```python
from build123d import *

# Parameters (mm, degrees)
SKETCH_1_W          = 55
SKETCH_1_H          = 40
EXTRUDE_1_DEPTH     = 13
SHELL_1_T           = -1
CHAMFER_1_SIZE      = 1
CUT_EXTRUDE_3_DEPTH = 2
EXTRUDE_5_DEPTH     = 12
SKETCH_16_W         = 5
SKETCH_16_H         = 11
CUT_EXTRUDE_4_DEPTH = 1
SKETCH_18_W         = 8
SKETCH_18_H         = 8
CUT_EXTRUDE_5_DEPTH = 10
SKETCH_19_W         = 1
SKETCH_19_H         = 8
EXTRUDE_6_DEPTH     = 1
SKETCH_21_W         = 0.2
SKETCH_21_H         = 1
CUT_EXTRUDE_6_DEPTH = 12
SKETCH_20_W         = 1.5
SKETCH_20_H         = 10
EXTRUDE_8_DEPTH     = 17.5
EXTRUDE_9_DEPTH     = 10
SKETCH_7_R          = 1
EXTRUDE_4_DEPTH     = 3
FILLET_1_R          = 2
FILLET_2_R          = 0.3
FILLET_3_R          = 0.3


with BuildPart() as part:
    # 草图1 → 凸台-拉伸1 (new body)
    with BuildSketch(Plane(origin=(0, 0, 0), x_dir=(1, 0, 0), z_dir=(0, 1, 0))):
        Rectangle(SKETCH_1_W, SKETCH_1_H)
    extrude(amount=EXTRUDE_1_DEPTH)

    # 抽壳1
    shell_1_openings = [part.faces().sort_by_distance(p)[0] for p in [
        (0, 0, 0),
    ]]
    offset(amount=SHELL_1_T, openings=shell_1_openings, kind=Kind.INTERSECTION)

    # 倒角1
    chamfer_1_edges = [part.edges().sort_by_distance(p)[0] for p in [
        (27.5, 13, 0),
        (0, 13, -20),
        (-27.5, 13, 0),
        (0, 13, 20),
        (-27.5, 6.5, -20),
        (27.5, 6.5, -20),
        (27.5, 6.5, 20),
        (-27.5, 6.5, 20),
    ]]
    chamfer(chamfer_1_edges, length=CHAMFER_1_SIZE)

    # 草图4 → 切除-拉伸3 (cut)
    with BuildSketch(Plane(origin=(27.5, 0, 0), x_dir=(0, 0, -1), z_dir=(1, 0, 0))):
        with BuildLine():
            Line((1.5, 4), (7.5, 4))
            ThreePointArc((7.5, 4), (9, 2.5), (7.5, 1))
            Line((7.5, 1), (1.5, 1))
            ThreePointArc((1.5, 1), (0, 2.5), (1.5, 4))
        make_face()
    extrude(amount=-CUT_EXTRUDE_3_DEPTH, mode=Mode.SUBTRACT)

    # 草图12 → 凸台-拉伸5 (add)
    with BuildSketch(Plane.XZ):
        with BuildLine():
            Line((26.5, -19), (23.5, -19))
            ThreePointArc((23.5, -19), (24.12244212, -16.62244212), (26.5, -16))
            Line((26.5, -16), (26.5, -19))
        make_face()
        with BuildLine():
            Line((-26.5, 19), (-23.5, 19))
            ThreePointArc((-23.5, 19), (-24.12244212, 16.62244212), (-26.5, 16))
            Line((-26.5, 16), (-26.5, 19))
        make_face()
    extrude(amount=-EXTRUDE_5_DEPTH)

    # 草图16 → 切除-拉伸4 (cut)
    with BuildSketch(Plane(origin=(0, 13, 0), x_dir=(1, 0, 0), z_dir=(0, 1, 0))):
        with Locations((-24, -7.69336468)):
            Rectangle(SKETCH_16_W, SKETCH_16_H)
    extrude(amount=-CUT_EXTRUDE_4_DEPTH, mode=Mode.SUBTRACT)

    # 草图18 → 切除-拉伸5 (cut)
    with BuildSketch(Plane.ZY.offset(27.5)):
        with Locations((-7, 4)):
            Rectangle(SKETCH_18_W, SKETCH_18_H)
    extrude(amount=-CUT_EXTRUDE_5_DEPTH, mode=Mode.SUBTRACT)

    # 草图19 → 凸台-拉伸6 (add)
    with BuildSketch(Plane(origin=(-26.5, 0, 0), x_dir=(0, 0, -1), z_dir=(1, 0, 0))):
        with Locations((2.5, 4)):
            Rectangle(SKETCH_19_W, SKETCH_19_H)
        with Locations((11.5, 4)):
            Rectangle(SKETCH_19_W, SKETCH_19_H)
    extrude(amount=EXTRUDE_6_DEPTH)

    # 草图21 → 切除-拉伸6 (cut)
    with BuildSketch(Plane.XZ):
        with Locations((-25.6, -11.5)):
            Rectangle(SKETCH_21_W, SKETCH_21_H)
        with Locations((-25.6, -2.5)):
            Rectangle(SKETCH_21_W, SKETCH_21_H)
    extrude(amount=-CUT_EXTRUDE_6_DEPTH, mode=Mode.SUBTRACT)

    # 草图20 → 凸台-拉伸8 (add)
    with BuildSketch(Plane.XZ.offset(-12)):
        with Locations((-24.25, -7)):
            Rectangle(SKETCH_20_W, SKETCH_20_H)
    extrude(amount=EXTRUDE_8_DEPTH)

    # 草图22 → 凸台-拉伸9 (add)
    with BuildSketch(Plane(origin=(0, 0, -12), x_dir=(-1, 0, 0), z_dir=(0, 0, -1))):
        Polygon((25, -5.5), (26.5, -4), (26.5, -3), (25, -3), align=None)
    extrude(amount=-EXTRUDE_9_DEPTH)

    # 草图7 → 凸台-拉伸4 (add)
    with BuildSketch(Plane.XZ):
        with Locations(Location((-25.5, 18, 0), (0, 0, 90))):
            Circle(SKETCH_7_R)
        with Locations(Location((25.5, -18, 0), (0, 0, 90))):
            Circle(SKETCH_7_R)
    extrude(amount=EXTRUDE_4_DEPTH)

    # 圆角1
    # the kernel refuses this fillet: 2 mm, written as the material it adds along each edge
    with BuildSketch(Plane(origin=(-25, 12, -12), x_dir=(-1, 0, 0), z_dir=(0, 0, 1)), Plane(origin=(-23.5, 12, -2), x_dir=(1, 0, 0), z_dir=(0, 0, -1))) as fillet_1_piece_1:
        with BuildLine():
            CenterArc((FILLET_1_R, FILLET_1_R), FILLET_1_R, 180, 90)
            Line((0, FILLET_1_R), (0, 0))
            Line((0, 0), (FILLET_1_R, 0))
        make_face()
    extrude(amount=10)

    # 圆角2
    fillet_2_edges = [part.edges().sort_by_distance(p)[0] for p in [
        (-25, -5.5, -7),
        (-24.25, -5.5, -12),
        (-23.5, -5.5, -7),
        (-24.25, -5.5, -2),
        (-25, -3, -7),
        (-26.5, -3, -7),
        (-26.5, -4, -7),
        (-25.75, -4.75, -12),
        (-25.75, -4.75, -2),
    ]]
    fillet(fillet_2_edges, radius=FILLET_2_R)

    # 圆角3
    fillet_3_edges = [part.edges().sort_by_distance(p)[0] for p in [
        (-27.5, 0, 8),
        (-27.5, 4, -11),
        (-27.5, 4, -3),
        (-26.6, 0, -3),
        (-26.6, 0, -11),
        (-27.5, 0, -15),
        (0, 0, -20),
        (27.5, 0, 0),
        (0, 0, 20),
    ]]
    fillet(fillet_3_edges, radius=FILLET_3_R)


solid = part.part
```
Check sheet for the modelled part. Datum: model origin and axes. Units: mm. A direction names the side the tool comes from. Give positions to 0.01 mm unless a question says otherwise; leave off trailing zeros. Order: outer loops, then holes, each group sorted by start corner. A loop starts at its lowest first (then second) coordinate and runs counter-clockwise, first axis right, second up. Notation, with made-up numbers: M -20.75,-22 L -5.75,-22 A36 cw -5.75,17 Z; hole C 44.25,-2.75 d3. An arc over 180 degrees is marked long. Answer in a Markdown table with one row per item. Add a question column.
Q1. Access from +Z, -Z, +X, -X, +Y, -Y to the whole of each face (thin tool, end or side, straight path). Record for faces 4 (the cylindrical face through (-25.4, 11.2, -7.1)), 5 (the flat face through (-24, -5.5, -7)), 6 (the cylindrical face through (27, 2.5, 0)), 7 (the flat face through (-24, 3, -2)).
Q2. Sectioned sample at C-C, the plane y = 2.5. Count the separate pieces of the cut face and the enclosed holes in it, and give its area (3 significant figures).
Q3. Sectioned sample at B-B, the plane z = 9. Record the boundary of the cut face in (x, y), and give its area (3 significant figures).
Q4. Thickness scan on L1, parallel to Z at x = -4, y = 2.5; L2, parallel to X at y = 5.25, z = -13; L3, parallel to X at y = 4.5, z = -11.5. Record the ranges inside material, lowest first.
Q5. Sectioned sample at D-D, the plane x = -7.5. Record the boundary of the cut face in (y, z).
Q6. Release check for a two-part mould opening along X. For faces 1 (the cylindrical face through (24.097, 5.916, -16.648)), 2 (the cylindrical face through (-24.61, -1.48, 18.46)), 3 (the cylindrical face through (27, 2.5, -9)) record: released by +X, released by -X, zero draft, split by the parting line, or undercut.
Q7. Sectioned sample at A-A, the plane y = 9. Record the boundary of the cut face in (x, z), and give its area (3 significant figures).
Q8. Gauge pin test, flat ends, axial feed: pin 1 Ø2 at (x, z) = (-4.5, 5.5) entering from -Y; pin 2 Ø1 at (x, z) = (26, -18.5) entering from -Y; pin 3 Ø0.8 at (x, z) = (27, -5.5) entering from -Y. Record the tip position at first contact, or that the pin passes through.
Verdict:
| question | item | result |
|---|---|---|
| 1 | face 4 | none |
| 1 | face 5 | +Z, -Z, +X, -X, -Y |
| 1 | face 6 | +X |
| 1 | face 7 | -Y |
| 2 | separate pieces | 3 |
| 2 | enclosed holes | 0 |
| 2 | area | 200 mm² |
| 3 | outline | M -27.5,0.3 A0.3 ccw -27.2,0 L -26.5,0 L -26.5,13 L -27.5,12 Z; M -21.5,12 L 26.5,12 L 26.5,0 L 27.2,0 A0.3 ccw 27.5,0.3 L 27.5,12 L 26.5,13 L -21.5,13 Z |
| 3 | area | 73.0 mm² |
| 4 | L1 | -20 to -19, 19 to 20 |
| 4 | L2 | -27.5 to -26.5, 26.5 to 27.5 |
| 4 | L3 | -27.5 to -25.7, -25 to -23.5, 26.5 to 27.5 |
| 5 | outline | M 0,-19.7 A0.3 ccw 0.3,-20 L 12,-20 L 13,-19 L 13,19 L 12,20 L 0.3,20 A0.3 ccw 0,19.7 L 0,19 L 12,19 L 12,-19 L 0,-19 Z |
| 6 | face 1 | undercut |
| 6 | face 2 | split by the parting line |
| 6 | face 3 | zero draft |
| 7 | outline | M -27.5,-19 L -26.5,-20 L 26.5,-20 L 27.5,-19 L 27.5,19 L 26.5,20 L -26.5,20 L -27.5,19 Z; M -25,-12 L -23.5,-12 L -23.5,-2 L -25,-2 Z; hole M -26.5,-19 L 23.5,-19 A2.43 cw 26.5,-16 L 26.5,19 L -23.5,19 A2.43 cw -26.5,16 Z |
| 7 | area | 215 mm² |
| 8 | pin 1 | y = 12 |
| 8 | pin 2 | y = -3 |
| 8 | pin 3 | y = 0 |
